from build123d import *

# Parameters (mm, degrees)
EXTRUDE_1_DEPTH = 2


with BuildPart() as part:
    # Model → 凸台-拉伸1 (new body)
    with BuildSketch(Plane.XY):
        with BuildLine():
            Line((13.756138035, 8.504570041), (154.085282898, 9.270484114))
            Line((154.085282898, 9.270484114), (155.225675402, 18.558235729))
            Line((155.225675402, 18.558235729), (153.736856174, 18.741039745))
            Line((153.736856174, 18.741039745), (154.930535969, 28.462781514))
            ThreePointArc((154.930535969, 28.462781514), (151.455462166, 22.111002891), (145.226629731, 18.420084836))
            Line((145.226629731, 18.420084836), (62.369712658, 17.275299877))
            ThreePointArc((62.369712658, 17.275299877), (56.144799442, 20.522983318), (53.589360421, 27.062610501))
            Line((53.589360421, 27.062610501), (52.370666987, 17.137148984))
            Line((52.370666987, 17.137148984), (50.881847759, 17.319952999))
            Line((50.881847759, 17.319952999), (52.075527554, 27.041694768))
            ThreePointArc((52.075527554, 27.041694768), (48.600453751, 20.689916146), (42.371621316, 16.998998091))
            Line((42.371621316, 16.998998091), (26.265146572, 16.776464467))
            ThreePointArc((26.265146572, 16.776464467), (20.040233356, 20.024147907), (17.484794335, 26.56377509))
            Line((17.484794335, 26.56377509), (16.266100901, 16.638313574))
            Line((16.266100901, 16.638313574), (14.777281674, 16.821117589))
            Line((14.777281674, 16.821117589), (13.756138035, 8.504570041))
        make_face()
    extrude(amount=EXTRUDE_1_DEPTH)


solid = part.part
Design review of the part built by this model. Coordinates are the model's own, in mm. A direction names the side the tool comes from. Round coordinates to 2 decimals unless told otherwise and drop trailing zeros. Write each loop counter-clockwise with the first axis right and the second up, starting at its lowest first coordinate (ties: lowest second). Pieces come first, ordered by that corner, then holes. Notation, with made-up numbers: M 77.25,-5.5 L 109.25,-5.5 A14 ccw 109.25,19.5 Z; hole C -13.75,85 d4. An arc over 180 degrees is marked long. One line per item, written item: value. Start each with the question number.
1. Draft analysis for pull direction X (two halves, no side actions). For faces 3 (the face through (151.53, 22.19, 0.99)), 4 (the face through (84, 14, 0)), state which applies: pulls with the +X half, pulls with the -X half, needs draft (parallel to the pull), parting line crosses it, or undercut.
2. Take a section at A-A on y = 23. State the section outline as (x, z) points, then the cut area to 3 significant figures.
3. To check wall thickness, follow probe 1 along X at (y, z) = (22.5, 1.8); probe 2 along X at (y, z) = (24.75, 0.3); probe 3 along Y at (x, z) = (98.5, 1.1). State the ranges of each line that lie inside material, in increasing order. Write a range as from..to.
4. Take a section at D-D on x = 29. State the section outline as (y, z) points.
5. Clearance check with flat-ended pins moving along their axes: P1, Ø1, axis at y = 24.5, z = 0.5, coming from the -X side; P2, Ø1, axis at y = 17, z = 1, coming from the +X side. State where each tip first meets the part, or that it passes through.
6. For faces 1 (the face through (56.21, 20.45, 0.99)), 2 (the face through (84, 14, 2)), list the 3-axis set-ups (+Z, -Z, +X, -X, +Y, -Y) from which the entire face can be reached by the end or side of a thin tool; tool diameter is ignored.
7. Take a section at C-C on x = 106.5. State the section outline as (y, z) points, then the cut area to 3 significant figures.
8. Take a section at B-B on z = 1. State the section outline as (x, y) points, then the cut area to 3 significant figures.
Computed:
1. face 3: undercut
1. face 4: needs draft
2. outline: M 17.05,0 L 18.19,0 L 18.19,2 L 17.05,2 Z; M 50.4,0 L 51.58,0 L 51.58,2 L 50.4,2 Z; M 53.09,0 L 54.51,0 L 54.51,2 L 53.09,2 Z; M 152.24,0 L 154.26,0 L 154.26,2 L 152.24,2 Z
2. area: 11.5 mm²
3. probe 1: x = 16.99..18.41, 50.07..51.52, 53.03..54.76, 151.82..154.2
3. probe 2: x = 17.26..17.68, 51.31..51.79, 53.31..53.89, 153.45..154.47
3. probe 3: y = 8.97..17.77
4. outline: M 8.59,0 L 16.81,0 L 16.81,2 L 8.59,2 Z
5. P1: stops at x = 17.17
5. P2: stops at x = 155.1
6. face 1: +Z, -Z, +Y
6. face 2: +Z, +X, -X, +Y, -Y
7. outline: M 9.01,0 L 17.89,0 L 17.89,2 L 9.01,2 Z
7. area: 17.7 mm²
8. outline: M 13.76,8.5 L 154.09,9.27 L 155.23,18.56 L 153.74,18.74 L 154.93,28.46 A13.69 cw 145.23,18.42 L 62.37,17.28 A10 cw 53.59,27.06 L 52.37,17.14 L 50.88,17.32 L 52.08,27.04 A13.69 cw 42.37,17 L 26.27,16.78 A10 cw 17.48,26.56 L 16.27,16.64 L 14.78,16.82 Z
8. area: 1,320 mm²
